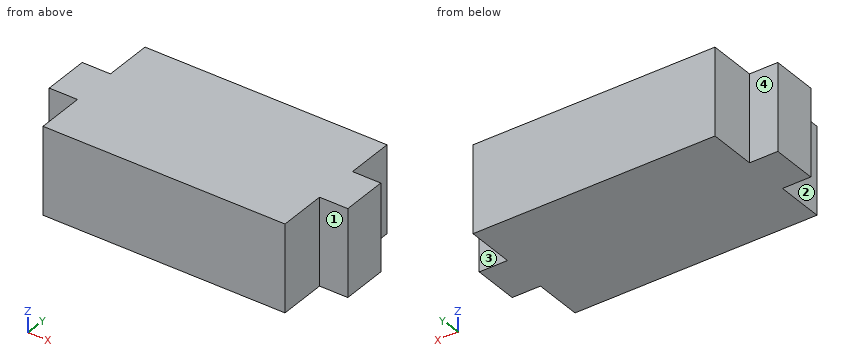
```python
from build123d import *

# Parameters (mm, degrees)
F0_W     = 8.255
F0_H     = 13.335
F1_DEPTH = 12.7


with BuildPart() as f1:
    # F0 (on Top) → F1 (new body, symmetric)
    with BuildSketch(Plane.XY):
        Polygon((35.306, 6.6675), (35.306, 20.6375), (-35.306, 20.6375), (-35.306, 6.6675), (-35.306, -6.6675), (-35.306, -20.6375), (35.306, -20.6375), (35.306, -6.6675), align=None)
        with Locations((-39.4335, 0)):
            Rectangle(F0_W, F0_H)
        with Locations((39.4335, 0)):
            Rectangle(F0_W, F0_H)
    extrude(amount=F1_DEPTH, both=True)


solid = f1.part
```
Can you work these out from the model? Positions are in its coordinate system, mm. Face numbers are marked on the shaded views. A direction names the side the tool comes from. Give positions to 0.01 mm unless a question says otherwise; leave off trailing zeros. Loops run counter-clockwise (first coordinate to the right, second up) from the corner with the lowest first, then second, coordinate; pieces in that order, holes last. Notation, with made-up numbers: M 60,-26.75 L 103,-26.75 A21 ccw 103,-16.75 Z; hole C 79.25,19 d1. An arc over 180 degrees is marked long. One line per item, written item: value.
(1) Suppose I cut it at A-A on z = -5.25. List the corners of the cut face in (x, y) for me.
Returned:
outline: M -43.56,-6.67 L -35.31,-6.67 L -35.31,-20.64 L 35.31,-20.64 L 35.31,-6.67 L 43.56,-6.67 L 43.56,6.67 L 35.31,6.67 L 35.31,20.64 L -35.31,20.64 L -35.31,6.67 L -43.56,6.67 Z
(2) Which directions (+Z, -Z, +X, -X, +Y, -Y) give clear straight access to the entire face, cutting with the end or side of a thin tool? Please do the marked faces 1, 2, 3 and 4.
Returned:
face 1: +Z, -Z, +X, -Y
face 2: +Z, -Z, -X, -Y
face 3: +Z, -Z, +X, +Y
face 4: +Z, -Z, -X, +Y
(3) I need wall thicknesses on line 1 (X direction, y = -12, z = -6.25); line 2 (Y direction, x = 40, z = -4.75). Which ranges of each line are inside material? Lowest first, please.
Returned:
line 1: -35.31 to 35.31
line 2: -6.67 to 6.67
(4) Suppose I cut it at B-B on y = 8. List the corners of the cut face in (x, z) for me.
Returned:
outline: M -35.31,-12.7 L 35.31,-12.7 L 35.31,12.7 L -35.31,12.7 Z
(5) Will these pins go through, and if not, where does the flat tip stop? pin 1 (9 mm diameter, centred on x = 38, z = -5, fed in from +Y); pin 2 (7 mm diameter, centred on y = -12, z = 3.5, fed in from +X); pin 3 (4 mm diameter, centred on x = 37.5, z = 3, fed in from -Y); pin 4 (2.5 mm diameter, centred on x = -41, z = 6.5, fed in from +Y).
Returned:
pin 1: y = 20.64
pin 2: x = 35.31
pin 3: y = -6.67
pin 4: y = 6.67
